Read the model definition and answer for the solid it produces. Units are mm, in the model's axes. A direction names the side the tool comes from. Round coordinates to 2 decimals unless told otherwise and drop trailing zeros. Order: outer loops, then holes, each group sorted by start corner. A loop starts at its lowest first (then second) coordinate and runs counter-clockwise, first axis right, second up. Notation, with made-up numbers: (40.25, 19) -> (49.25, 19) arc R26 ccw to (49.25, 44) -> close; hole circle Ø9 at (26, -29). An arc over 180 degrees is marked (long way). Use a Markdown table: item, result. Add a question column.
1. Section D-D, the plane z = 10 is taken. Give the vertices of the cut face in (x, y).
2. Section A-A, the plane y = 53 is taken. Give the vertices of the cut face in (x, z), then the cut area to 3 significant figures.
3. The mould has two halves that part along X. Classify faces 4 (the face through (90.909, -6.156, 3.131)), 5 (the face through (-51.42, -6.06, 3.13)), 6 (the face through (-41, 11, 3.81)): +X half, -X half, draft (parallel to the pull), parting line (faces both ways), or undercut.
4. Section C-C, the plane z = 21.75 is taken. Give the vertices of the cut face in (x, y), then the cut area to 3 significant figures.
5. Consider L1, parallel to X at y = 11, z = 5; L2, parallel to Z at x = -9, y = 19; L3, parallel to Z at x = 30, y = 27.5. Determine where each line is inside the solid, lowest interval first. Write a range as [from, to].
6. For faces 1 (the face through (-41, 17, 5.715)), 2 (the face through (24.98, 26.02, 12.83)), 3 (the face through (91.01, 59.97, 3.13)), determine the directions among +Z, -Z, +X, -X, +Y, -Y from which every point of the face is accessible in a straight line to the end or side of a thin tool.
7. Section B-B, the plane x = -9 is taken. Give the vertices of the cut face in (y, z).
8. Given pin 1 (1.5 mm diameter, centred on y = 27.5, z = 9, fed in from +X); pin 2 (8 mm diameter, centred on y = 25, z = 14, fed in from -X); pin 3 (1 mm diameter, centred on x = -31.5, y = 8, fed in from +Z); pin 4 (6 mm diameter, centred on y = 54, z = 6.5, fed in from -X), each flat-ended and moving along its own axis, determine where each tip first touches the part or whether it passes through.
```python
from build123d import *

# Parameters (mm, degrees)
F1_DEPTH = 6.35
F3_DEPTH = 2.54
F4_R     = 3.175
F4_R_2   = 1.5875
F5_DEPTH = 1.905
F6_R     = 0.635
F7_DEPTH = 1.27
F8_R     = 19.05
F9_DEPTH = 1.27


with BuildPart() as f1:
    # F0 (on Top) → F1 (new body)
    with BuildSketch(Plane.XY):
        with BuildLine():
            Line((86.468494, 61.882985), (-46.881506, 61.882985))
            ThreePointArc((-46.881506, 61.882985), (-51.371634, 60.023113), (-53.231506, 55.532985))
            Line((-53.231506, 55.532985), (-53.231506, -1.617015))
            ThreePointArc((-53.231506, -1.617015), (-51.371634, -6.107143), (-46.881506, -7.967015))
            Line((-46.881506, -7.967015), (86.468494, -7.967015))
            ThreePointArc((86.468494, -7.967015), (90.958622, -6.107143), (92.818494, -1.617015))
            Line((92.818494, -1.617015), (92.818494, 55.532985))
            ThreePointArc((92.818494, 55.532985), (90.958622, 60.023113), (86.468494, 61.882985))
        make_face()
    extrude(amount=F1_DEPTH)

    # F2 (on face) → F3 (cut)
    with BuildSketch(Plane.XY.offset(6.35)):
        with BuildLine():
            ThreePointArc((-46.881506, 4.732985), (-45.021634, 0.242857), (-40.531506, -1.617015))
            Line((-40.531506, -1.617015), (-36.721506, -1.617015))
            ThreePointArc((-36.721506, -1.617015), (-34.925455, -0.873067), (-34.181506, 0.922985))
            Line((-34.181506, 0.922985), (-34.181506, 17.432985))
            ThreePointArc((-34.181506, 17.432985), (-36.041378, 21.923113), (-40.531506, 23.782985))
            Line((-40.531506, 23.782985), (-44.341506, 23.782985))
            ThreePointArc((-44.341506, 23.782985), (-46.137557, 23.039036), (-46.881506, 21.242985))
            Line((-46.881506, 21.242985), (-46.881506, 4.732985))
        make_face()
    extrude(amount=-F3_DEPTH, mode=Mode.SUBTRACT)

    # F4 (on face) → F5 (join)
    with BuildSketch(Plane.XY.offset(3.81)):
        with Locations((-40.531506, 4.732985)):
            Circle(F4_R)
        with Locations((-40.531506, 17.432985)):
            Circle(F4_R_2)
    extrude(amount=F5_DEPTH)

    # F6 (on face) → F7 (join)
    with BuildSketch(Plane.XY.offset(3.81)):
        with Locations((-40.258363, 11.830621)):
            Circle(F6_R)
    extrude(amount=F7_DEPTH)

    # F8 (on face) → F9 (join)
    with BuildSketch(Plane.XY.offset(6.35)):
        with Locations((19.793494, 26.957985)):
            Circle(F8_R)
    extrude(amount=F9_DEPTH)

    # F11 (on offset) → F12 (revolve)
    with BuildSketch(Plane.YZ.offset(19.304)):
        Polygon((27.2852, 25.904429), (27.2852, 6.854429), (45.8272, 25.904429), align=None)
    revolve(axis=Axis((19.304, 27.2852, 16.379429), (0, 0, 1)))


solid = f1.part
```
Verdict:
| question | item | result |
|---|---|---|
| 1 | outline | circle Ø6.12 at (19.3, 27.29) |
| 2 | outline | (-53.23, 0) -> (92.82, 0) -> (92.82, 6.35) -> (-53.23, 6.35) -> close |
| 2 | area | 927 mm2 |
| 3 | face 4 | +X half |
| 3 | face 5 | -X half |
| 3 | face 6 | undercut |
| 4 | outline | circle Ø29 at (19.3, 27.29) |
| 4 | area | 660 mm2 |
| 5 | L1 | x = [-53.23, -46.88], [-34.18, 92.82] |
| 5 | L2 | z = [0, 6.35] |
| 5 | L3 | z = [0, 7.62], [17.85, 25.9] |
| 6 | face 1 | +Z |
| 6 | face 2 | none |
| 6 | face 3 | +Z, -Z, +X, +Y |
| 7 | outline | (-7.97, 0) -> (61.88, 0) -> (61.88, 6.35) -> (-7.97, 6.35) -> close |
| 8 | pin 1 | stops at x = 22.12 |
| 8 | pin 2 | stops at x = 8.63 |
| 8 | pin 3 | stops at z = 6.35 |
| 8 | pin 4 | stops at x = -53.23 |
